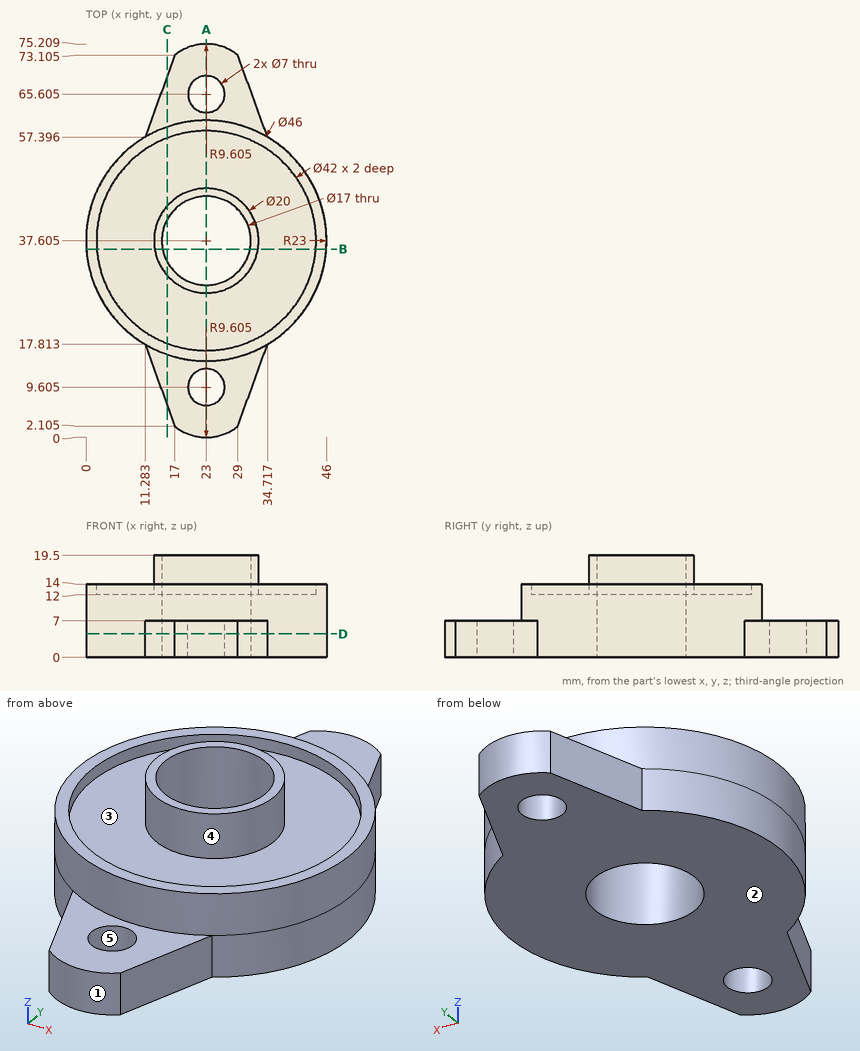
Answer from the drawing. Dimensions are ordinates in mm from the lowest x, y and z of the part. A direction names the side the tool comes from. Coordinates: 2 decimals unless noted, no trailing zeros. Loops run counter-clockwise (first coordinate to the right, second up) from the corner with the lowest first, then second, coordinate; pieces in that order, holes last. Notation, with made-up numbers: (21.5, 20.5) -> (47.5, 20.5) arc R20 ccw to (47.5, 51.5) -> close; hole circle Ø3 at (12, 3.25). An arc over 180 degrees is marked (long way). Answer in a Markdown table with one row per item.
Item 1: A cutting plane is placed at C-C on x = 15.5. Determine the outline of the cut face in (y, z) (1 decimal).
Returned:
| item | result |
|---|---|
| outline | (6.2, 0) -> (33.6, 0) -> (33.6, 19.5) -> (31, 19.5) -> (31, 12) -> (18, 12) -> (18, 14) -> (15.9, 14) -> (15.9, 7) -> (6.2, 7) -> close; (41.6, 0) -> (69, 0) -> (69, 7) -> (59.3, 7) -> (59.3, 14) -> (57.2, 14) -> (57.2, 12) -> (44.2, 12) -> (44.2, 19.5) -> (41.6, 19.5) -> close |
Item 2: A cutting plane is placed at A-A on x = 23. Determine the outline of the cut face in (y, z) (1 decimal).
Returned:
| item | result |
|---|---|
| outline | (0, 0) -> (6.1, 0) -> (6.1, 7) -> (0, 7) -> close; (13.1, 0) -> (29.1, 0) -> (29.1, 19.5) -> (27.6, 19.5) -> (27.6, 12) -> (16.6, 12) -> (16.6, 14) -> (14.6, 14) -> (14.6, 7) -> (13.1, 7) -> close; (46.1, 0) -> (62.1, 0) -> (62.1, 7) -> (60.6, 7) -> (60.6, 14) -> (58.6, 14) -> (58.6, 12) -> (47.6, 12) -> (47.6, 19.5) -> (46.1, 19.5) -> close; (69.1, 0) -> (75.2, 0) -> (75.2, 7) -> (69.1, 7) -> close |
Item 3: A cutting plane is placed at B-B on y = 36. Determine the outline of the cut face in (x, z).
Returned:
| item | result |
|---|---|
| outline | (0.06, 0) -> (14.65, 0) -> (14.65, 19.5) -> (13.13, 19.5) -> (13.13, 12) -> (2.06, 12) -> (2.06, 14) -> (0.06, 14) -> close; (31.35, 0) -> (45.94, 0) -> (45.94, 14) -> (43.94, 14) -> (43.94, 12) -> (32.87, 12) -> (32.87, 19.5) -> (31.35, 19.5) -> close |
Item 4: For a pull along Y with two mould halves and no side action, classify the marked faces 1, 2 and 3 as released by +Y, released by -Y, zero draft, split by the parting line, or undercut.
Returned:
| item | result |
|---|---|
| face 1 | released by -Y |
| face 2 | zero draft |
| face 3 | undercut |
Item 5: For the marked faces 4 and 5, determine the directions among +Z, -Z, +X, -X, +Y, -Y from which every point of the face is accessible in a straight line to the end or side of a thin tool.
Returned:
| item | result |
|---|---|
| face 4 | +Z |
| face 5 | +Z, -Z |
Item 6: Each of these flat-tipped pins is pushed along its axis until it touches: P1, Ø5.5, axis at x = 23, y = 9.6, coming from the -Z side; P2, Ø6, axis at y = 57, z = 7, coming from the -X side; P3, Ø1, axis at x = 17, z = 4, coming from the -Y side; P4, Ø6, axis at x = 39.5, z = 10.5, coming from the -Y side. Where does it stop, or does it pass through?
Returned:
| item | result |
|---|---|
| P1 | passes through |
| P2 | stops at x = 6.87 |
| P3 | stops at y = 1.73 |
| P4 | stops at y = 18.98 |
Item 7: A cutting plane is placed at D-D on z = 4.5. Determine the outline of the cut face in (x, y) (1 decimal).
Returned:
| item | result |
|---|---|
| outline | (11.3, 17.8) -> (17, 2.1) arc R9.6 ccw to (29, 2.1) -> (34.7, 17.8) arc R23 ccw to (34.7, 57.4) -> (29, 73.1) arc R9.6 ccw to (17, 73.1) -> (11.3, 57.4) arc R23 ccw to start; hole circle Ø17 at (23, 37.6); hole circle Ø7 at (23, 9.6); hole circle Ø7 at (23, 65.6) |
Item 8: Straight lines are drawn through the part: line 1 along Y through (x, z) = (23, 12.75) (1 decimal); line 2 along Y through (x, z) = (23, 1.5) (1 decimal); line 3 along Z through (x, y) = (33, 15.5). For each, find the intervals that lie inside material, in ascending order. Write a range as [from, to].
Returned:
| item | result |
|---|---|
| line 1 | y = [14.6, 16.6], [27.6, 29.1], [46.1, 47.6], [58.6, 60.6] |
| line 2 | y = [0, 6.1], [13.1, 29.1], [46.1, 62.1], [69.1, 75.2] |
| line 3 | z = [0, 7] |
